```python
from build123d import *

# Parameters (mm, degrees)
BOSS_EXTRU_1_DEPTH      = 40
ESQUISSE2_R             = 12.5
ENL_V_MAT_EXTRU_1_DEPTH = 945.245730729
CONG_1_R                = 20
ENL_V_MAT_EXTRU_4_DEPTH = 945.245730729


with BuildPart() as part:
    # Esquisse1 → Boss.-Extru.1 (new body)
    with BuildSketch(Plane.XY):
        Polygon((500, 0), (500, 800), (-300, 700), (-300, 100), align=None)
    extrude(amount=BOSS_EXTRU_1_DEPTH)

    # Esquisse2 → Enlèv. mat.-Extru.1 (cut, through all)
    with BuildSketch(Plane(origin=(0, 0, 0), x_dir=(1, 0, 0), z_dir=(0, 1, 0))):
        with Locations((460, -20)):
            Circle(ESQUISSE2_R)
    extrude(amount=ENL_V_MAT_EXTRU_1_DEPTH, mode=Mode.SUBTRACT)

    # Congé1
    cong_1_edges = [part.edges().sort_by_distance(p)[0] for p in [
        (-300, 400, 0),
        (-300, 400, 40),
        (500, 400, 0),
        (500, 400, 40),
    ]]
    fillet(cong_1_edges, radius=CONG_1_R - 0.0001)  # a hair under: the kernel refuses the full size

    # Esquisse3 → Enlèv. mat.-Extru.4 (cut, through all)
    with BuildSketch(Plane.XY):
        Polygon((-300, 639.533066888), (-300, 160.466933112), (-292.557915925, 159.536672603), (-272.557915925, 157.036672603), (420, 70.466933112), (420, 729.533066888), (-272.557915925, 642.963327397), (-292.557915925, 640.463327397), align=None)
    extrude(amount=ENL_V_MAT_EXTRU_4_DEPTH, mode=Mode.SUBTRACT)


solid = part.part
```
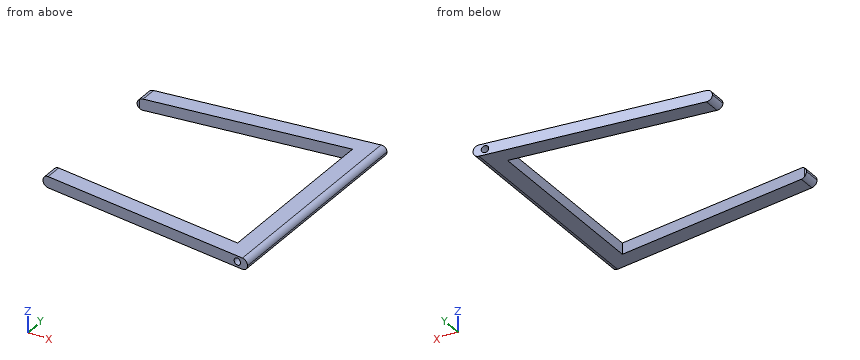
CAD build for the part. Positions are in the model's coordinates, mm. Round coordinates to 2 decimals unless told otherwise and drop trailing zeros. Order: outer loops, then holes, each group sorted by start corner. A loop starts at its lowest first (then second) coordinate and runs counter-clockwise, first axis right, second up. Notation, with made-up numbers: (59, 70) - (118, 70) arc R17 ccw to (118, 93) - close; hole circle Ø9 at (-39.75, -23.5). An arc over 180 degrees is marked (long way). Answer in a Markdown table with one row per item. Add a question column.
(1) Band-saw the part on C-C on x = -141. List the corners of the cut face in (y, z) (3 decimals).
(2) Probe L1, parallel to Z at x = 460, y = 227; L2, parallel to X at y = 427, z = 19.5; L3, parallel to Y at x = -208.5, z = 30. List the from-to ranges inside material, lowest first. Write a range as [from, to].
(3) Band-saw the part on A-A on x = 460. List the corners of the cut face in (y, z).
(4) Drop flat-ended pins along their axis: pin 1 Ø5 at (x, z) = (237.5, 23) entering from -Y; pin 2 Ø20 at (y, z) = (496.5, 27) entering from -X; pin 3 Ø1.5 at (y, z) = (381, 34) entering from +X. Give the stop position or say it passes through.
Data:
| question | item | result |
|---|---|---|
| 1 | outline | (80.125, 0) - (140.592, 0) - (140.592, 40) - (80.125, 40) - close; (659.408, 0) - (719.875, 0) - (719.875, 40) - (659.408, 40) - close |
| 2 | L1 | z = [0, 7.5], [32.5, 40] |
| 2 | L2 | x = [420, 447.51], [472.49, 499.99] |
| 2 | L3 | y = [88.56, 149.03], [650.97, 711.44] |
| 3 | outline | (5, 0) - (795, 0) - (795, 7.5) - (5, 7.5) - close; (5, 32.5) - (795, 32.5) - (795, 40) - (5, 40) - close |
| 4 | pin 1 | stops at y = 32.5 |
| 4 | pin 2 | stops at x = 420 |
| 4 | pin 3 | stops at x = 494.98 |
